Can you work these out from the drawing? Everything is in mm from the part's minimum corner. Coordinates: 2 decimals unless noted, no trailing zeros. Loops run counter-clockwise (first coordinate to the right, second up) from the corner with the lowest first, then second, coordinate; pieces in that order, holes last.
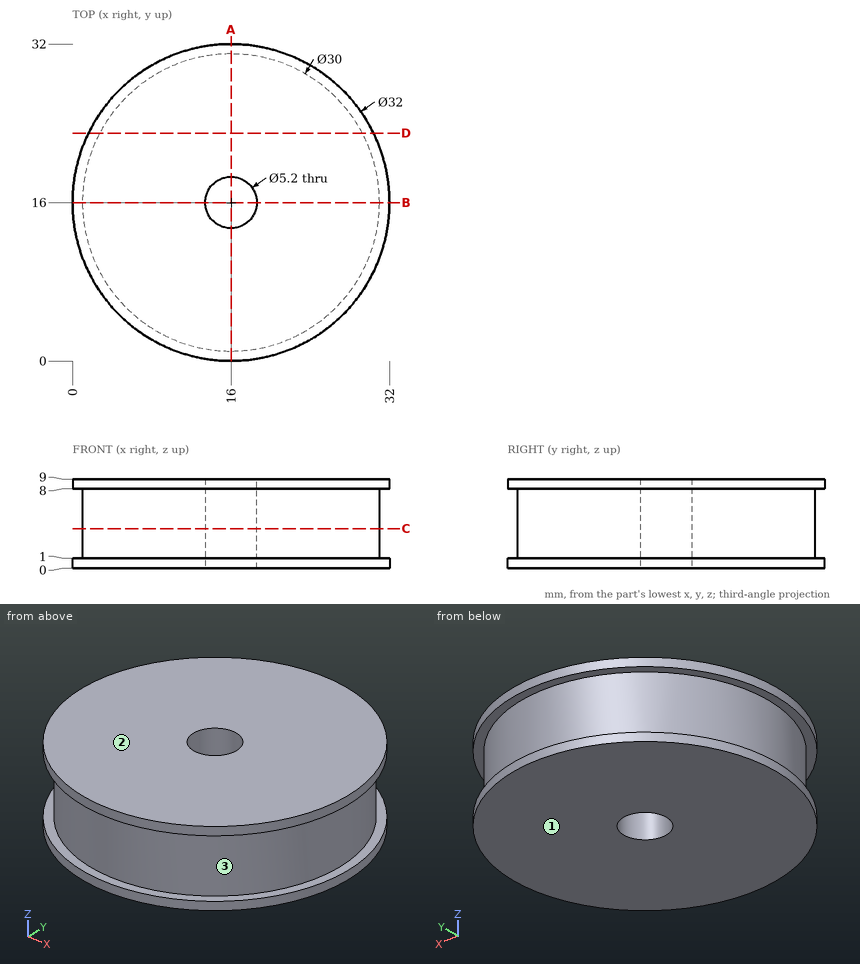
(1) We'd pull the mould along Z, two halves only. Please class the marked faces 1, 2 and 3: +Z half, -Z half, draft (parallel to the pull), parting line (faces both ways), or undercut.
Answers:
face 1: -Z half
face 2: +Z half
face 3: undercut
(2) Imagine slicing it at A-A, the plane x = 16. Write out the boundary of the cut face in (y, z), and give its area (3 significant figures).
Answers:
outline: (0, 0) - (13.4, 0) - (13.4, 9) - (0, 9) - (0, 8) - (1, 8) - (1, 1) - (0, 1) - close; (18.6, 0) - (32, 0) - (32, 1) - (31, 1) - (31, 8) - (32, 8) - (32, 9) - (18.6, 9) - close
area: 227 mm2
(3) Imagine slicing it at D-D, the plane y = 23. Write out the boundary of the cut face in (x, z), and give its area (3 significant figures).
Answers:
outline: (1.61, 0) - (30.39, 0) - (30.39, 1) - (29.27, 1) - (29.27, 8) - (30.39, 8) - (30.39, 9) - (1.61, 9) - (1.61, 8) - (2.73, 8) - (2.73, 1) - (1.61, 1) - close
area: 243 mm2
(4) For pin 1 (1 mm diameter, centred on y = 9, z = 3, fed in from +X); pin 2 (3 mm diameter, centred on y = 18.5, z = 1.5, fed in from +X); pin 3 (5 mm diameter, centred on x = 28, z = 6.5, fed in from -Y), each with a flat end and sliding along its axis, tell me the tip position at first contact or that it passes through.
Answers:
pin 1: stops at x = 29.52
pin 2: stops at x = 31.96
pin 3: stops at y = 3.51
(5) Imagine slicing it at C-C, the plane z = 4. Write out the boundary of the cut face in (x, y), and give its area (3 significant figures).
Answers:
outline: circle Ø30 at (16, 16); hole circle Ø5.2 at (16, 16)
area: 686 mm2
(6) I need wall thicknesses on probe 1 along Y at (x, z) = (16, 2.75); probe 2 along Z at (x, y) = (30.5, 21.5); probe 3 along X at (y, z) = (18, 5). Which ranges of each line are inside material? Lowest first, please.
Answers:
probe 1: y = 1 to 13.4, 18.6 to 31
probe 2: z = 0 to 1, 8 to 9
probe 3: x = 1.13 to 14.34, 17.66 to 30.87
